Here's the drawing with two shaded views (mm, measured from the low corner). I have some questions. A direction names the side the tool comes from. Coordinates: 2 decimals unless noted, no trailing zeros. Order: outer loops, then holes, each group sorted by start corner. A loop starts at its lowest first (then second) coordinate and runs counter-clockwise, first axis right, second up. Notation, with made-up numbers: (-39, 83.5) - (4, 83.5) arc R24 ccw to (4, 102.5) - close; hole circle Ø2 at (-12.5, 83). An arc over 180 degrees is marked (long way). Answer as CSV lines item,"result". Start each with the question number.
1. I need wall thicknesses on probe 1 along Z at (x, y) = (26.25, 27.4); probe 2 along X at (y, z) = (26.5, 1.5); probe 3 along Z at (x, y) = (37, 2.55). Which ranges of each line are inside material? Lowest first, please.
2. I want a section at B-B, the plane y = 20. List the corners of the cut face in (x, z) for me.
3. I want a section at A-A, the plane x = 5. List the corners of the cut face in (y, z) for me, and give its area (3 significant figures).
4. Thinking about a two-plate mould opening in X: for the marked faces 4, 5 and 6, which applies, released by +X, released by -X, zero draft, split by the parting line, or undercut?
5. I want a section at D-D, the plane y = 27.4. List the corners of the cut face in (x, z) for me, and give its area (3 significant figures).
6. For pin 1 (4 mm diameter, centred on y = 30.5, z = 3.5, fed in from +X); pin 2 (4 mm diameter, centred on y = 29, z = 3.5, fed in from -X); pin 3 (3.5 mm diameter, centred on x = 8, z = 7.5, fed in from +Y), each with a flat end and sliding along its axis, tell me the tip position at first contact or that it passes through.
7. I want a section at C-C, the plane z = 11.5. List the corners of the cut face in (x, y) for me.
8. For the marked faces 1, 2 and 3, which set-ups out of +Z, -Z, +X, -X, +Y, -Y let a thin tool reach every point of the face, with its end or its side?
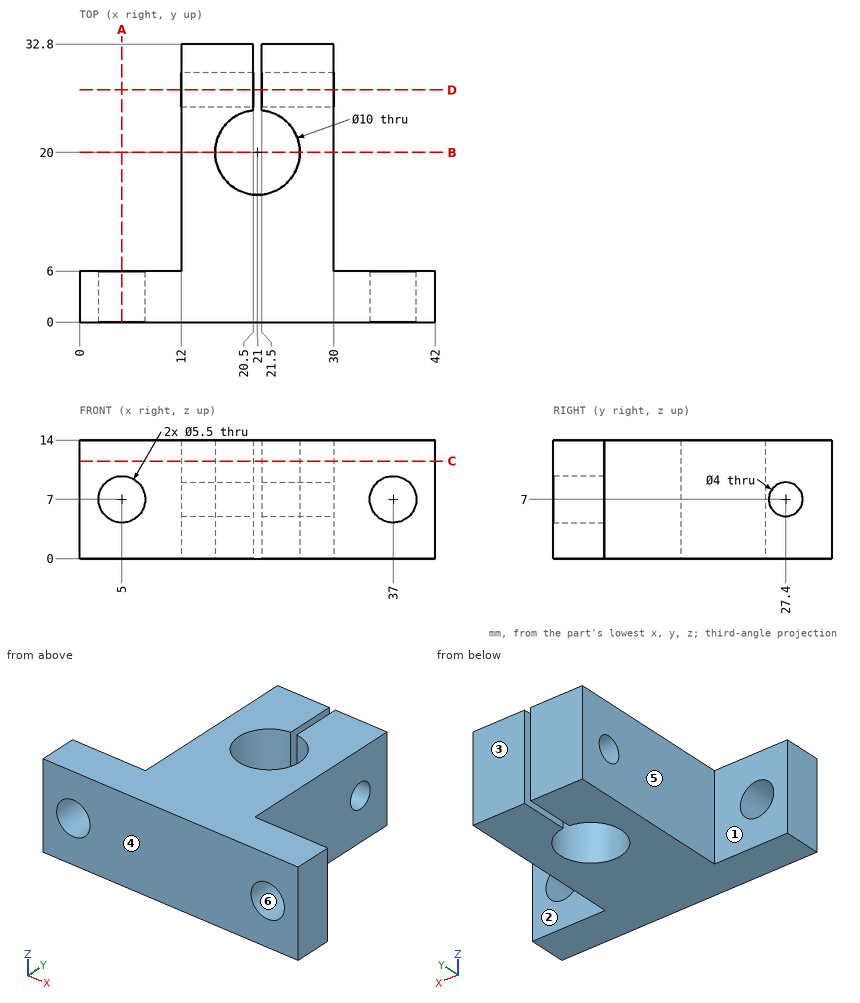
Solved:
1,probe 1,"z = 0 to 5, 9 to 14"
1,probe 2,"x = 12 to 20.5, 21.5 to 30"
1,probe 3,"z = 0 to 4.25, 9.75 to 14"
2,outline,"(12, 0) - (16, 0) - (16, 14) - (12, 14) - close; (26, 0) - (30, 0) - (30, 14) - (26, 14) - close"
3,outline,"(0, 0) - (6, 0) - (6, 4.25) - (0, 4.25) - close; (0, 9.75) - (6, 9.75) - (6, 14) - (0, 14) - close"
3,area,"51.0 mm2"
4,face 4,"zero draft"
4,face 5,"released by -X"
4,face 6,"undercut"
5,outline,"(12, 0) - (20.5, 0) - (20.5, 5) - (12, 5) - close; (12, 9) - (20.5, 9) - (20.5, 14) - (12, 14) - close; (21.5, 0) - (30, 0) - (30, 5) - (21.5, 5) - close; (21.5, 9) - (30, 9) - (30, 14) - (21.5, 14) - close"
5,area,"170 mm2"
6,pin 1,"stops at x = 30"
6,pin 2,"stops at x = 12"
6,pin 3,"stops at y = 6"
7,outline,"(0, 0) - (42, 0) - (42, 6) - (30, 6) - (30, 32.8) - (21.5, 32.8) - (21.5, 24.97) arc R5 cw (long way) to (20.5, 24.97) - (20.5, 32.8) - (12, 32.8) - (12, 6) - (0, 6) - close"
8,face 1,"+Z, -Z, -X, +Y"
8,face 2,"+Z, -Z, +X, +Y"
8,face 3,"+Z, -Z, +X, -X, +Y"
